Check sheet for the modelled part. Datum: model origin and axes. Units: mm. Face numbers are marked on the shaded views. A direction names the side the tool comes from. Round coordinates to 2 decimals unless told otherwise and drop trailing zeros. Write each loop counter-clockwise with the first axis right and the second up, starting at its lowest first coordinate (ties: lowest second). Pieces come first, ordered by that corner, then holes. Notation, with made-up numbers: M -39.5,50.25 L 7.5,50.25 A25 cw 7.5,69.25 Z; hole C 75.5,69 d11. An arc over 180 degrees is marked long. One line per item, written item: value.
from build123d import *

# Parameters (mm, degrees)
CROQUIS1_R              = 1
SALIENTE_EXTRUIR1_DEPTH = 1.7
CROQUIS3_W              = 15
CROQUIS3_H              = 10.99
SALIENTE_EXTRUIR2_DEPTH = 3.4
CROQUIS4_W              = 15
CROQUIS4_H              = 3.4
CORTAR_EXTRUIR1_DEPTH   = 10.99
SALIENTE_EXTRUIR3_DEPTH = 3.4


with BuildPart() as part:
    # Croquis1 → Saliente-Extruir1 (new, symmetric)
    with BuildSketch(Plane.XY):
        with BuildLine():
            Line((-3.6, 0), (-3.6, -10))
            ThreePointArc((-3.6, -10), (-2.545584412, -12.545584412), (0, -13.6))
            Line((0, -13.6), (28.6, -13.6))
            Line((28.6, -13.6), (28.6, -8.6))
            Line((28.6, -8.6), (23.6, -5))
            Line((23.6, -5), (3.6, -5))
            Line((3.6, -5), (3.6, 0))
            ThreePointArc((3.6, 0), (0, 3.6), (-3.6, 0))
        make_face()
        Circle(CROQUIS1_R, mode=Mode.SUBTRACT)
        with Locations((0, -10)):
            Circle(CROQUIS1_R, mode=Mode.SUBTRACT)
    extrude(amount=SALIENTE_EXTRUIR1_DEPTH, both=True)

    # Croquis3 → Saliente-Extruir2 (add)
    with BuildSketch(Plane(origin=(0, 0, -1.7), x_dir=(-1, 0, 0), z_dir=(0, 0, -1))):
        with Locations((-21.1, -19.095)):
            Rectangle(CROQUIS3_W, CROQUIS3_H)
    extrude(amount=-SALIENTE_EXTRUIR2_DEPTH)

    # Croquis4 → Cortar-Extruir1 (cut)
    with BuildSketch(Plane.XZ.offset(24.59)):
        with Locations((21.1, 0)):
            Rectangle(CROQUIS4_W, CROQUIS4_H)
    extrude(amount=-CORTAR_EXTRUIR1_DEPTH, mode=Mode.SUBTRACT)

    # Croquis5 → Saliente-Extruir3 (add)
    with BuildSketch(Plane.XY.offset(1.7)):
        with BuildLine():
            Line((28.6, -13.6), (28.6, -16.3))
            Line((28.6, -16.3), (-3.6, -16.3))
            Line((-3.6, -16.3), (-3.6, -10))
            ThreePointArc((-3.6, -10), (-2.545584412, -12.545584412), (0, -13.6))
            Line((0, -13.6), (28.6, -13.6))
        make_face()
    extrude(amount=-SALIENTE_EXTRUIR3_DEPTH)


solid = part.part
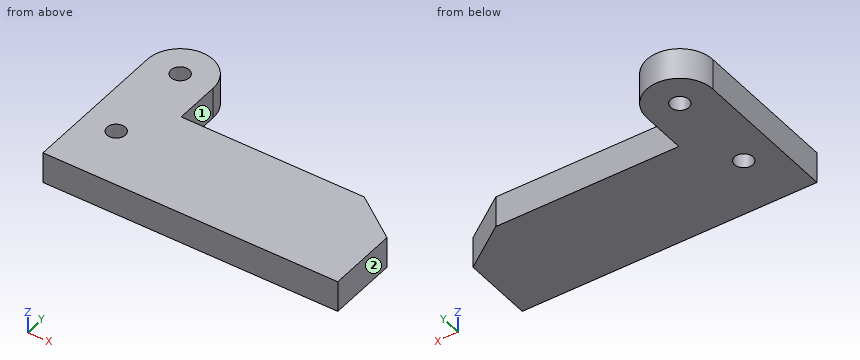
Q1. Scan lines: line 1 (Y direction, x = 0, z = -0.25); line 2 (X direction, y = -0.25, z = -0.85); line 3 (Y direction, x = 8, z = 1.4). Record each from-to range of solid material in increasing order. Write a range as [from, to].
Completed:
line 1: [-16.3, -11], [-9, -1], [1, 3.6]
line 2: [-3.6, -0.97], [0.97, 3.6]
line 3: [-16.3, -5]
Q2. Sectioned sample at D-D on y = -2. Enter the section's corners in (x, z), and give its area (3 significant figures).
Completed:
outline: M -3.6,-1.7 L 3.6,-1.7 L 3.6,1.7 L -3.6,1.7 Z
area: 24.5 mm^2
Q3. Sectioned sample at B-B on z = -0.45. Enter the section's corners in (x, y), and give its area (3 significant figures).
Completed:
outline: M -3.6,-16.3 L 28.6,-16.3 L 28.6,-8.6 L 23.6,-5 L 3.6,-5 L 3.6,0 A3.6 ccw -3.6,0 Z; hole C 0,-10 d2; hole C 0,0 d2
area: 405 mm^2
Q4. Access from +Z, -Z, +X, -X, +Y, -Y to the whole of each face (thin tool, end or side, straight path). Record for the marked faces 1 and 2.
Completed:
face 1: +Z, -Z, +X, +Y
face 2: +Z, -Z, +X, +Y, -Y
Q5. Sectioned sample at C-C on x = 0. Enter the section's corners in (y, z).
Completed:
outline: M -16.3,-1.7 L -11,-1.7 L -11,1.7 L -16.3,1.7 Z; M -9,-1.7 L -1,-1.7 L -1,1.7 L -9,1.7 Z; M 1,-1.7 L 3.6,-1.7 L 3.6,1.7 L 1,1.7 Z
Q6. Sectioned sample at A-A on y = -10. Enter the section's corners in (x, z), and give its area (3 significant figures).
Completed:
outline: M -3.6,-1.7 L -1,-1.7 L -1,1.7 L -3.6,1.7 Z; M 1,-1.7 L 28.6,-1.7 L 28.6,1.7 L 1,1.7 Z
area: 103 mm^2
Q7. Depth check by flat-ended pin: P1, Ø1, axis at y = -3.5, z = 0, coming from the +X side. Enter the tip coordinate at first touch or a pass-through.
Completed:
P1: x = 3.6
